from build123d import *

# Parameters (mm, degrees)
SKETCH1_W                   = 40
SKETCH1_H                   = 10
BOSS_EXTRUDE1_DEPTH         = 10
TAP_DRILL_FOR_M3X0_5_TAP1_D = 2.5


with BuildPart() as part:
    # Sketch1 → Boss-Extrude1 (new body)
    with BuildSketch(Plane.XY):
        Rectangle(SKETCH1_W, SKETCH1_H)
    extrude(amount=BOSS_EXTRUDE1_DEPTH)

    # Tap Drill for M3x0.5 Tap1 (through all)
    with Locations(Plane(origin=(0, -5, 0), x_dir=(-1, 0, 0), z_dir=(0, -1, 0))):
        with Locations((16, -5), (-16, -5)):
            Hole(TAP_DRILL_FOR_M3X0_5_TAP1_D / 2)


solid = part.part
Source: CAD feature listing. Evaluate the final solid. Frame: model axes, mm. Round coordinates to 2 decimals unless told otherwise and drop trailing zeros. Loops run counter-clockwise (first coordinate to the right, second up) from the corner with the lowest first, then second, coordinate; pieces in that order, holes last. Notation, with made-up numbers: M 4,-24 L 58,-24 A18 ccw 58,-17 Z; hole C -8,-6.5 d1. An arc over 180 degrees is marked long. Answer as CSV lines item,"result".
Q1. Line query: line 1 along X through (y, z) = (1.25, 5); line 2 along Z through (x, y) = (-16, -3); line 3 along X through (y, z) = (4, 4.5). Output: solid intervals per line, ascending.
Verdict:
line 1,"x = -20 to -17.25, -14.75 to 14.75, 17.25 to 20"
line 2,"z = 0 to 3.75, 6.25 to 10"
line 3,"x = -20 to -17.15, -14.85 to 14.85, 17.15 to 20"
Q2. Cut plane C-C (y = -1.25). Return the cut outline in (x, z).
Verdict:
outline,"M -20,0 L 20,0 L 20,10 L -20,10 Z; hole C -16,5 d2.5; hole C 16,5 d2.5"
Q3. Cut plane A-A (z = 5). Return the cut outline in (x, y).
Verdict:
outline,"M -20,-5 L -17.25,-5 L -17.25,5 L -20,5 Z; M -14.75,-5 L 14.75,-5 L 14.75,5 L -14.75,5 Z; M 17.25,-5 L 20,-5 L 20,5 L 17.25,5 Z"
Q4. Cut plane D-D (x = -16.5). Return the cut outline in (y, z), plus the area to 3 significant figures.
Verdict:
outline,"M -5,0 L 5,0 L 5,3.85 L -5,3.85 Z; M -5,6.15 L 5,6.15 L 5,10 L -5,10 Z"
area,"77.1 mm^2"
Q5. Cut plane B-B (x = 16). Return the cut outline in (y, z).
Verdict:
outline,"M -5,0 L 5,0 L 5,3.75 L -5,3.75 Z; M -5,6.25 L 5,6.25 L 5,10 L -5,10 Z"
Q6. Pull-direction query (Z, two-part tool) for faces 1 (the face through (0, 0, 0)), 2 (the face through (15.73, 0.07, 6.22)), 3 (the face through (0, 0, 10)), 4 (the face through (0, -5, 5)); classes: +Z half, -Z half, draft (parallel to the pull), parting line (faces both ways), or undercut.
Verdict:
face 1,"-Z half"
face 2,"undercut"
face 3,"+Z half"
face 4,"draft"
